from build123d import *

# Parameters (mm, degrees)
SKETCH1_R           = 12.600000000000001
BOSS_EXTRUDE1_DEPTH = 2.5
BOSS_EXTRUDE3_DEPTH = 2.5
SKETCH4_R           = 1.2499999999999973
SKETCH4_R_2         = 2.5000000000000018
SKETCH4_R_3         = 3.7
BOSS_EXTRUDE4_DEPTH = 2.5
CUT_EXTRUDE1_START  = -0.8333333333333334
SKETCH5_R           = 2.249999999999998
SKETCH5_R_2         = 1.2499999999999973
SKETCH5_R_3         = 2.500000000000002
SKETCH5_R_4         = 3.7
SKETCH5_R_5         = 2.2499999999999987
CUT_EXTRUDE1_DEPTH  = 0.8333333333333334
CHAMFER1_SIZE       = 0.5
CHAMFER2_SIZE       = 0.5
FILLET2_R           = 15
CHAMFER6_SIZE       = 6
CHAMFER6_SIZE2      = 10.392304845413321


with BuildPart() as part:
    # Sketch1 → Boss-Extrude1 (new, symmetric)
    with BuildSketch(Plane.XY):
        with BuildLine():
            Line((-17.5, -22.500000000000004), (-7.500000000000002, -22.500000000000004))
            Line((-7.500000000000002, -22.500000000000004), (-7.500000000000002, -16.5))
            Line((-7.500000000000002, -16.5), (7.500000000000005, -16.5))
            Line((7.500000000000005, -16.5), (7.500000000000007, -22.500000000000004))
            Line((7.500000000000007, -22.500000000000004), (17.500000000000007, -22.5))
            Line((17.500000000000007, -22.5), (17.500000000000004, 0))
            ThreePointArc((17.500000000000004, 0), (-2.81e-15, 17.500000000000004), (-17.500000000000004, -6.94e-15))
            Line((-17.500000000000004, -6.94e-15), (-17.5, -22.500000000000004))
        make_face()
        Circle(SKETCH1_R, mode=Mode.SUBTRACT)
    extrude(amount=BOSS_EXTRUDE1_DEPTH, both=True)

    # Sketch3 → Boss-Extrude3 (add, symmetric)
    with BuildSketch(Plane.XY):
        Polygon((17.500000000000007, -10.000000000000002), (17.500000000000004, 0), (32.70000000000001, 0), (32.70000000000001, -10), align=None)
    extrude(amount=BOSS_EXTRUDE3_DEPTH, both=True)

    # Sketch4 → Boss-Extrude4 (add)
    with BuildSketch(Plane(origin=(0, 0, -2.5), x_dir=(-1, 0, 0), z_dir=(0, 0, -1))):
        with BuildLine():
            Line((5.8309518948453105, -16.5), (-5.8309518948453105, -16.5))
            ThreePointArc((-5.8309518948453105, -16.5), (4.96e-15, 17.500000000000004), (5.8309518948453105, -16.5))
        make_face()
        with Locations((-8.5, 0)):
            Circle(SKETCH4_R, mode=Mode.SUBTRACT)
        with Locations((8.5, 0)):
            Circle(SKETCH4_R, mode=Mode.SUBTRACT)
        with Locations((0, -8.5)):
            Circle(SKETCH4_R_2, mode=Mode.SUBTRACT)
        with Locations((0, 8.5)):
            Circle(SKETCH4_R_2, mode=Mode.SUBTRACT)
        Circle(SKETCH4_R_3, mode=Mode.SUBTRACT)
    extrude(amount=BOSS_EXTRUDE4_DEPTH)

    # Sketch5 → Cut-Extrude1 (cut)
    # profile 1 of 3: a face of its own
    with BuildSketch(Plane(origin=(0, 0, -5), x_dir=(-1, 0, 0), z_dir=(0, 0, -1)).offset(CUT_EXTRUDE1_START)):
        with Locations((-8.5, 0)):
            Circle(SKETCH5_R)
        with Locations((-8.5, 0)):
            Circle(SKETCH5_R_2, mode=Mode.SUBTRACT)
    # profile 2 of 3: a face of its own
    with BuildSketch(Plane(origin=(0, 0, -5), x_dir=(-1, 0, 0), z_dir=(0, 0, -1)).offset(CUT_EXTRUDE1_START)):
        with BuildLine():
            Line((3.500000000000002, 8.5), (4.7, 0))
            Line((4.7, 0), (3.500000000000002, -8.5))
            ThreePointArc((3.500000000000002, -8.5), (-6.4e-16, -12.000000000000002), (-3.500000000000002, -8.5))
            Line((-3.500000000000002, -8.5), (-4.7, 0))
            Line((-4.7, 0), (-3.500000000000002, 8.5))
            ThreePointArc((-3.500000000000002, 8.5), (2.1e-16, 12.000000000000002), (3.500000000000002, 8.5))
        make_face()
        with Locations((0, 8.5)):
            Circle(SKETCH5_R_3, mode=Mode.SUBTRACT)
        with Locations((0, -8.5)):
            Circle(SKETCH5_R_3, mode=Mode.SUBTRACT)
        Circle(SKETCH5_R_4, mode=Mode.SUBTRACT)
    # profile 3 of 3: a face of its own
    with BuildSketch(Plane(origin=(0, 0, -5), x_dir=(-1, 0, 0), z_dir=(0, 0, -1)).offset(CUT_EXTRUDE1_START)):
        with Locations((8.5, 0)):
            Circle(SKETCH5_R_5)
        with Locations((8.5, 0)):
            Circle(SKETCH5_R_2, mode=Mode.SUBTRACT)
    extrude(amount=CUT_EXTRUDE1_DEPTH, mode=Mode.SUBTRACT)

    # Chamfer1
    chamfer1_edges = [part.edges().sort_by_distance(p)[0] for p in [
        (-2.66e-15, 17.500000000000004, -5),
        (0, -16.5, -5),
        (10.749999999999998, 2.8e-16, -5),
        (-4.100000000000001, 4.25, -5),
        (-4.100000000000001, -4.25, -5),
        (-1e-17, 12, -5),
        (4.100000000000001, 4.25, -5),
        (4.100000000000001, -4.25, -5),
        (2.3e-16, -12, -5),
        (-6.250000000000002, 2.8e-16, -5),
    ]]
    chamfer(chamfer1_edges, length=CHAMFER1_SIZE)

    # Chamfer2
    chamfer2_edges = [part.edges().sort_by_distance(p)[0] for p in [
        (-12.600000000000001, 1.54e-15, 2.5),
        (3.7, 4.5e-16, -2.5),
        (2.5000000000000018, 8.5, -2.5),
        (2.5000000000000018, -8.5, -2.5),
        (-7.250000000000003, 1.5e-16, -2.5),
        (9.749999999999996, 1.5e-16, -2.5),
    ]]
    chamfer(chamfer2_edges, length=CHAMFER2_SIZE)

    # Chamfer4
    # the kernel refuses this chamfer: 12 mm, written as the material it adds along each edge
    with BuildSketch(Plane(origin=(17.500000000000004, 0, 2.5), x_dir=(0.999648118666469, -0.026526191709121207, 0), z_dir=(0, 0, -1))) as chamfer4_piece_1:
        with BuildLine():
            Line((9.855061796439113, 1e-17), (-2.110948481595115, -7.326644011468382))
            Line((-2.110948481595115, -7.326644011468382), (-2.3275279701108307, -7.223235476258414))
            ThreePointArc((-2.3275279701108307, -7.223235476258414), (-0.7534896907076923, -3.7391476844990703), (-0.239915548479951, 0.00636628601018905))
            Line((-0.239915548479951, 0.00636628601018905), (0.00636628601018909, 0.23991554847995256))
            ThreePointArc((0.00636628601018909, 0.23991554847995256), (4.93042998207199, 0.10925291314792994), (9.861428082449303, 0.2399155484799526))
            Line((9.861428082449303, 0.2399155484799526), (9.855061796439113, 1e-17))
        make_face()
    extrude(amount=5)

    # Fillet2
    fillet2_edges = [part.edges().sort_by_distance(p)[0] for p in [
        (15.986710313133337, 7.118644067795235, 0),
    ]]
    fillet(fillet2_edges, radius=FILLET2_R)

    # Chamfer6
    chamfer6_edges = [part.edges().sort_by_distance(p)[0] for p in [
        (17.500000000000007, -10.000000000000002, 0),
    ]]
    chamfer6_side = [part.faces().sort_by_distance(p)[0] for p in [
        (17.500000000000007, -16.25, 4e-17),
    ]]
    chamfer(chamfer6_edges, length=CHAMFER6_SIZE, length2=CHAMFER6_SIZE2, reference=chamfer6_side[0])


solid = part.part
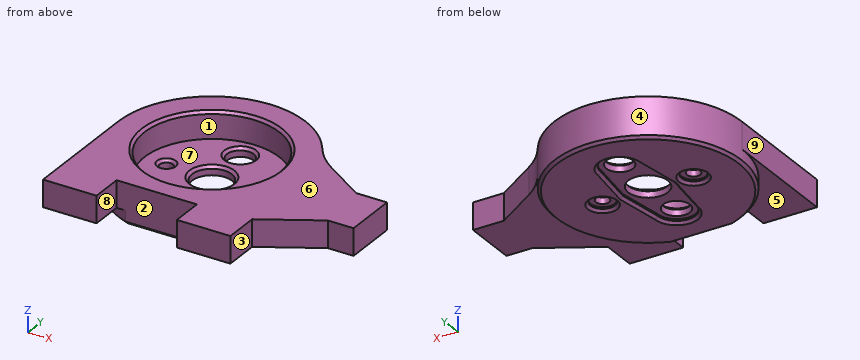
Work out the finished part from the listing and answer in its coordinate system (mm). Face numbers are marked on the shaded views. A direction names the side the tool comes from. Round coordinates to 2 decimals unless told otherwise and drop trailing zeros. Write each loop counter-clockwise with the first axis right and the second up, starting at its lowest first coordinate (ties: lowest second). Pieces come first, ordered by that corner, then holes. Notation, with made-up numbers: M -15,60.5 L 33,60.5 A25 ccw 33,75.5 Z; hole C 68,-6 d8. An arc over 180 degrees is marked long. Use a Markdown table: item, result.
1) Which of the six approach directions +Z, -Z, +X, -X, +Y, -Y give full straight-line access (tool end or side, diameter ignored) to the marked faces 1, 2, 3, 4 and 5?
Taken from the geometry:
| item | result |
|---|---|
| face 1 | +Z |
| face 2 | +Z, -Z, -Y |
| face 3 | +Z, -Z, +X, -Y |
| face 4 | -Z |
| face 5 | -Z, -X, -Y |
2) Determine the mould class of the marked faces 6, 7, 8 and 9 for opening direction X: pulls with the +X half, pulls with the -X half, needs draft (parallel to the pull), parting line crosses it, or undercut.
Taken from the geometry:
| item | result |
|---|---|
| face 6 | needs draft |
| face 7 | undercut |
| face 8 | undercut |
| face 9 | pulls with the -X half |
3) Consider line 1 (Y direction, x = 0, z = -3.7); line 2 (Y direction, x = 9.5, z = 1.75); line 3 (Y direction, x = -9.5, z = -3.25). Determine where each line is inside the solid, lowest interval first. Write a range as [from, to].
Taken from the geometry:
| item | result |
|---|---|
| line 1 | y = [-16.5, -11], [-6, -3.7], [3.7, 6], [11, 17.5] |
| line 2 | y = [-22.5, -8.28], [8.28, 14.7] |
| line 3 | y = [-14.7, -0.75], [0.75, 14.7] |
4) The part is cut by section A-A on z = -1. Give the vertices of the cut face in (x, y).
Taken from the geometry:
| item | result |
|---|---|
| outline | M -17.5,-22.5 L -7.5,-22.5 L -7.5,-16.5 L 7.5,-16.5 L 7.5,-22.5 L 17.5,-22.5 L 17.5,-16 L 27.89,-10 L 32.7,-10 L 32.7,0 L 26.95,0 L 19.1,5.09 A15 cw 14.69,9.52 A17.5 ccw -17.5,0 Z; hole C 0,0 d25.2 |
5) The part is cut by section B-B on x = 0. State how many separate pieces and enclosed holes the cut face has, plus the area to 3 significant figures.
Taken from the geometry:
| item | result |
|---|---|
| separate pieces | 4 |
| enclosed holes | 0 |
| area | 78.5 mm2 |
6) Flat-ended cylindrical pins translate along their axes: pin 1 (1.5 mm diameter, centred on x = 13.5, z = 0, fed in from +Y); pin 2 (2 mm diameter, centred on x = 2.5, z = 0, fed in from -Y); pin 3 (6 mm diameter, centred on x = 0, y = 0, fed in from -Z); pin 4 (8 mm diameter, centred on x = 0, y = 8.5, fed in from +Z). Find the tip coordinate at first contact, or state that the pin passes through.
Taken from the geometry:
| item | result |
|---|---|
| pin 1 | stops at y = 11.99 |
| pin 2 | stops at y = -16.5 |
| pin 3 | passes through |
| pin 4 | stops at z = -2.5 |
7) The part is cut by section C-C on x = 21. Give the vertices of the cut face in (y, z).
Taken from the geometry:
| item | result |
|---|---|
| outline | M -13.98,-2.5 L 3.86,-2.5 L 3.86,2.5 L -13.98,2.5 Z |
